Input: part model. Units: mm. Frame: model coordinates. A direction names the side the tool comes from. Round coordinates to 2 decimals unless told otherwise and drop trailing zeros. Loops run counter-clockwise (first coordinate to the right, second up) from the corner with the lowest first, then second, coordinate; pieces in that order, holes last. Notation, with made-up numbers: (-10.5, 61) -> (12.5, 61) arc R23 cw to (12.5, 87) -> close; hole circle Ø6 at (-25.75, 41). An arc over 180 degrees is marked (long way). Answer as a JSON object with one key per item and string values.
```python
from build123d import *

# Parameters (mm, degrees)
SKETCH1_W           = 21
SKETCH1_H           = 10
SKETCH2_R           = 18
CUT_EXTRUDE1_DEPTH  = 32.336879232
SKETCH4_R           = 19.4
BOSS_EXTRUDE1_DEPTH = 5
SKETCH5_R           = 18
CUT_EXTRUDE2_DEPTH  = 34.271609519


with BuildPart() as part:
    # Sketch1 → Revolve1 (revolve)
    with BuildSketch(Plane.XY, mode=Mode.PRIVATE) as revolve1_sk:
        with Locations((10.5, 5)):
            Rectangle(SKETCH1_W, SKETCH1_H)
    revolve(revolve1_sk.sketch.rotate(Axis((0, 0, 0), (0, 1, 0)), 90), axis=Axis((0, 0, 0), (0, 1, 0)))

    # Sketch2 → Cut-Extrude1 (cut, through all)
    with BuildSketch(Plane(origin=(0, 10, 0), x_dir=(1, 0, 0), z_dir=(0, 1, 0))):
        with Locations(Location((0, 0, 0), (0, 0, 270))):
            Circle(SKETCH2_R)
    extrude(amount=-CUT_EXTRUDE1_DEPTH, mode=Mode.SUBTRACT)

    # Sketch4 → Boss-Extrude1 (add)
    with BuildSketch(Plane(origin=(0, 10, 0), x_dir=(1, 0, 0), z_dir=(0, 1, 0))):
        with Locations(Location((0, 0, 0), (0, 0, 270))):
            Circle(SKETCH4_R)
    extrude(amount=BOSS_EXTRUDE1_DEPTH)

    # Sketch5 → Cut-Extrude2 (cut, through all)
    with BuildSketch(Plane(origin=(0, 15, 0), x_dir=(1, 0, 0), z_dir=(0, 1, 0))):
        with Locations(Location((0, 0, 0), (0, 0, 270))):
            Circle(SKETCH5_R)
    extrude(amount=-CUT_EXTRUDE2_DEPTH, mode=Mode.SUBTRACT)


solid = part.part
```
1) Contact query for flat-ended pins moving along their axis: P1, Ø4, axis at y = 8, z = 4, coming from the -X side; P2, Ø4, axis at x = -8, y = 4.5, coming from the +Z side; P3, Ø1.5, axis at y = 4, z = 13.5, coming from the -X side. Output: stop coordinate, or through.
Output:
{"P1": "stops at x = -20.9", "P2": "stops at z = 20.12", "P3": "stops at x = -16.69"}
2) Section A-A, the plane x = 0. Output: boundary loops of the cut face in (y, z).
Output:
{"outline": "(0, -21) -> (10, -21) -> (10, -19.4) -> (15, -19.4) -> (15, -18) -> (0, -18) -> close; (0, 18) -> (15, 18) -> (15, 19.4) -> (10, 19.4) -> (10, 21) -> (0, 21) -> close"}
3) Reachability of faces 1 (the face through (5.827, 12.465, 18.504)), 2 (the face through (-13, 15, 13)) from +Z, -Z, +X, -X, +Y, -Y: full face, straight path, thin tool, end or side. Return the list, or none.
Output:
{"face 1": "+Y", "face 2": "+Z, -Z, +X, -X, +Y"}
4) Section C-C, the plane y = 13.25. Output: boundary loops of the cut face in (x, z).
Output:
{"outline": "circle Ø38.8 at (0, 0); hole circle Ø36 at (0, 0)"}
5) Section B-B, the plane z = 0. Output: boundary loops of the cut face in (x, y).
Output:
{"outline": "(-21, 0) -> (-18, 0) -> (-18, 15) -> (-19.4, 15) -> (-19.4, 10) -> (-21, 10) -> close; (18, 0) -> (21, 0) -> (21, 10) -> (19.4, 10) -> (19.4, 15) -> (18, 15) -> close"}
6) Section D-D, the plane y = 9.5. Output: boundary loops of the cut face in (x, z), plus the area to 3 significant figures.
Output:
{"outline": "circle Ø42 at (0, 0); hole circle Ø36 at (0, 0)", "area": "368 mm^2"}
7) Draft query along X for faces 3 (the face through (5.407, 7.605, 17.169)), 4 (the face through (-16, 0, -9)), 5 (the face through (-6.31, 5.07, -20.03)). Return one class per face: +X half, -X half, draft (parallel to the pull), parting line (faces both ways), or undercut.
Output:
{"face 3": "undercut", "face 4": "draft", "face 5": "parting line"}
8) Ray query, probe 1 along X at (y, z) = (10.25, 0); probe 2 along X at (y, z) = (6, 0); probe 3 along Y at (x, z) = (-11, -16.5). Return the intervals inside material, ascending.
Output:
{"probe 1": "x = -19.4 to -18, 18 to 19.4", "probe 2": "x = -21 to -18, 18 to 21", "probe 3": "y = 0 to 10"}
